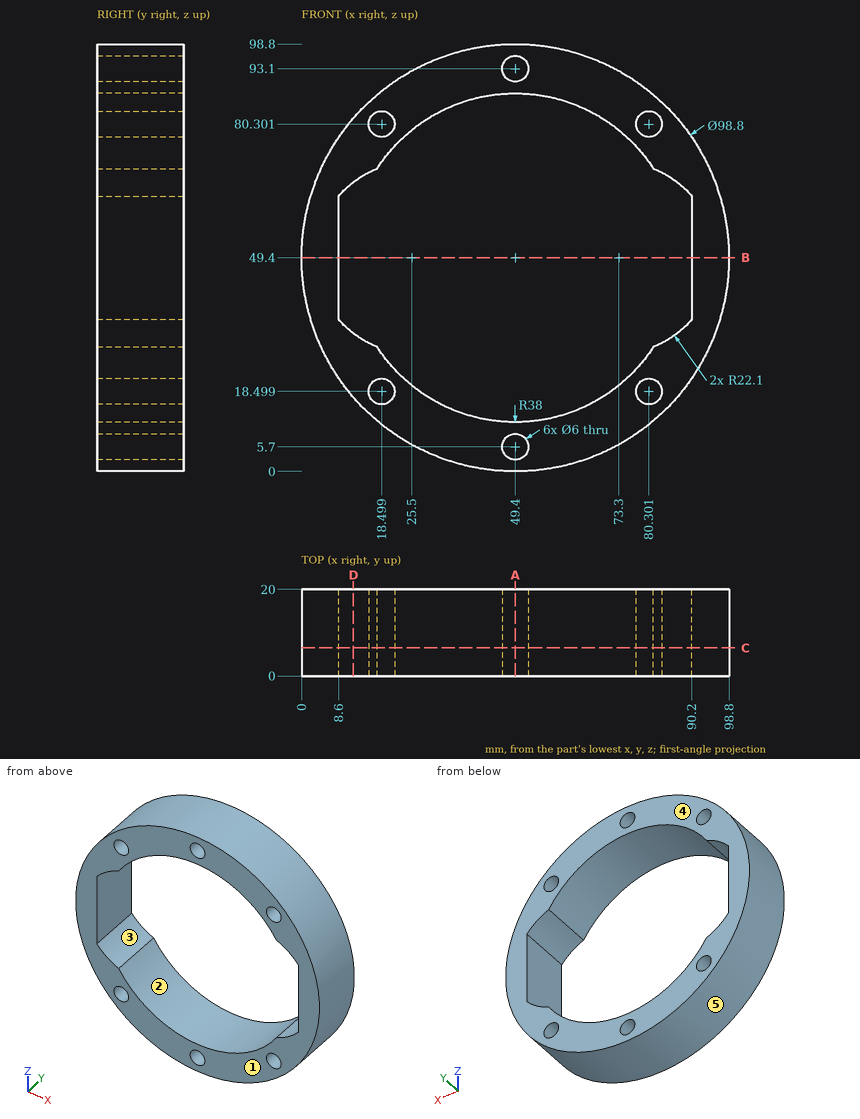
The drawing under review shows one solid part. Ordinate dimensions are in mm from its lowest x, y, z. A direction names the side the tool comes from. Round coordinates to 2 decimals unless told otherwise and drop trailing zeros. Loops run counter-clockwise (first coordinate to the right, second up) from the corner with the lowest first, then second, coordinate; pieces in that order, holes last.
Item 1: Take a section at C-C (y = 6.5). Write out the cut boundary in (x, z) (1 decimal), then the cut area to 3 significant figures.
Determined:
outline: circle Ø98.8 at (49.4, 49.4); hole (8.6, 35.2) arc R22.1 ccw to (17.5, 28.8) arc R38 ccw to (81.3, 28.8) arc R22.1 ccw to (90.2, 35.2) - (90.2, 63.6) arc R22.1 ccw to (81.3, 70) arc R38 ccw to (17.5, 70) arc R22.1 ccw to (8.6, 63.6) - close; hole circle Ø6 at (18.5, 18.5); hole circle Ø6 at (18.5, 80.3); hole circle Ø6 at (49.4, 5.7); hole circle Ø6 at (49.4, 93.1); hole circle Ø6 at (80.3, 18.5); hole circle Ø6 at (80.3, 80.3)
area: 2,660 mm2
Item 2: Mouldability with a two-part tool opening along X and no side actions: class the marked faces 3, 4 and 5 as released by +X, released by -X, zero draft, split by the parting line, or undercut.
Determined:
face 3: undercut
face 4: zero draft
face 5: split by the parting line
Item 3: Take a section at B-B (z = 49.4). Write out the cut boundary in (x, y).
Determined:
outline: (0, 0) - (8.6, 0) - (8.6, 20) - (0, 20) - close; (90.2, 0) - (98.8, 0) - (98.8, 20) - (90.2, 20) - close
Item 4: For the marked faces 1 and 2, list the 3-axis set-ups (+Z, -Z, +X, -X, +Y, -Y) from which the entire face can be reached by the end or side of a thin tool; tool diameter is ignored.
Determined:
face 1: +Z, -Z, +X, -X, -Y
face 2: +Y, -Y
Item 5: For line 1 (Z direction, x = 83, y = 16) (1 decimal); line 2 (X direction, y = 16, z = 19) (1 decimal); line 3 (X direction, y = 5, z = 49), list the stretches that pass through material, from the lowest coordinate up.
Determined:
line 1: z = 13.2 to 17.2, 19.8 to 29.5, 69.3 to 79, 81.6 to 85.6
line 2: x = 10.5 to 15.5, 21.5 to 26.6, 72.2 to 77.3, 83.3 to 88.3
line 3: x = 0 to 8.6, 90.2 to 98.8
Item 6: Take a section at D-D (x = 12). Write out the cut boundary in (y, z), then the cut area to 3 significant figures.
Determined:
outline: (0, 17.13) - (20, 17.13) - (20, 31.9) - (0, 31.9) - close; (0, 66.9) - (20, 66.9) - (20, 81.67) - (0, 81.67) - close
area: 591 mm2
Item 7: Take a section at A-A (x = 49.4). Write out the cut boundary in (y, z).
Determined:
outline: (0, 0) - (20, 0) - (20, 2.7) - (0, 2.7) - close; (0, 8.7) - (20, 8.7) - (20, 11.4) - (0, 11.4) - close; (0, 87.4) - (20, 87.4) - (20, 90.1) - (0, 90.1) - close; (0, 96.1) - (20, 96.1) - (20, 98.8) - (0, 98.8) - close
Item 8: Clearance check with flat-ended pins moving along their axes: pin 1 Ø4 at (x, y) = (40, 15.5) entering from +Z; pin 2 Ø5 at (x, z) = (18.5, 18.5) entering from +Y; pin 3 Ø1.5 at (y, z) = (3, 53.5) entering from +X; pin 4 Ø8 at (x, y) = (63.5, 12) entering from +Z. State where each tip first meets the part, or that it passes through.
Determined:
pin 1: stops at z = 98.24
pin 2: passes through
pin 3: stops at x = 98.69
pin 4: stops at z = 97.76
